Geometry check sheet. Reference: drawing and pictorial views, mm from the part's lowest x, y, z. A direction names the side the tool comes from. Give positions to 0.01 mm unless a question says otherwise; leave off trailing zeros. Order: outer loops, then holes, each group sorted by start corner. A loop starts at its lowest first (then second) coordinate and runs counter-clockwise, first axis right, second up. Notation, with made-up numbers: (-26, 61.25) - (25, 61.25) arc R29 cw to (25, 98.25) - close; hole circle Ø1 at (22, 46.5). An arc over 180 degrees is marked (long way). Answer as a JSON object with one key per item and string values.
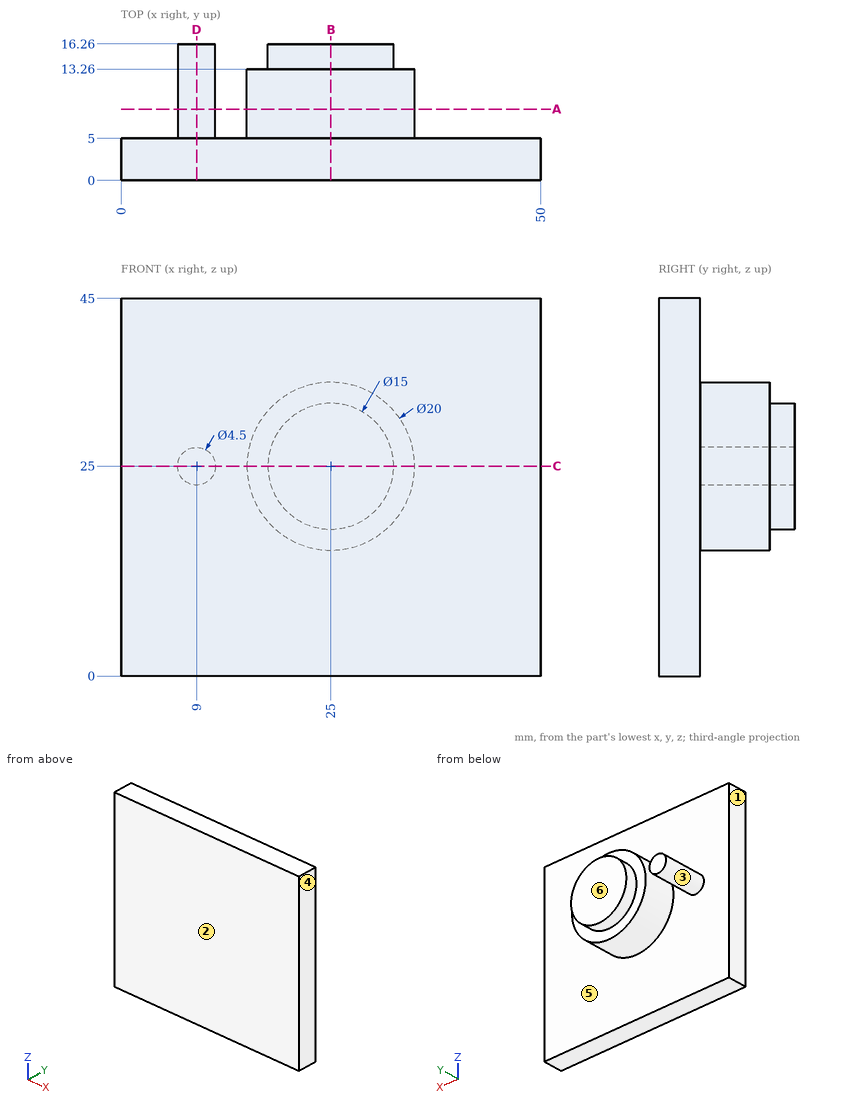
(1) Gauge pin test, flat ends, axial feed: pin 1 Ø6 at (x, y) = (35, 13) entering from -Z; pin 2 Ø1 at (x, y) = (8.5, 11) entering from +Z. Record the tip position at first contact, or that the pin passes through.
Computed values:
{"pin 1": "stops at z = 17.86", "pin 2": "stops at z = 27.25"}
(2) Section check B-B (x = 25). Record the cut outline in (y, z).
Computed values:
{"outline": "(0, 0) - (5, 0) - (5, 15) - (13.26, 15) - (13.26, 17.5) - (16.26, 17.5) - (16.26, 32.5) - (13.26, 32.5) - (13.26, 35) - (5, 35) - (5, 45) - (0, 45) - close"}
(3) Access from +Z, -Z, +X, -X, +Y, -Y to the whole of each face (thin tool, end or side, straight path). Record for the marked faces 5 and 6.
Computed values:
{"face 5": "+Y", "face 6": "+Z, -Z, +X, -X, +Y"}
(4) Section check C-C (z = 25). Record the cut outline in (x, y).
Computed values:
{"outline": "(0, 0) - (50, 0) - (50, 5) - (35, 5) - (35, 13.26) - (32.5, 13.26) - (32.5, 16.26) - (17.5, 16.26) - (17.5, 13.26) - (15, 13.26) - (15, 5) - (11.25, 5) - (11.25, 16.26) - (6.75, 16.26) - (6.75, 5) - (0, 5) - close"}
(5) Section check A-A (y = 8.5). Record the cut outline in (x, z).
Computed values:
{"outline": "circle Ø4.5 at (9, 25); circle Ø20 at (25, 25)"}
(6) Material ranges on line 1 along Y through (x, z) = (44.5, 43); line 2 along Y through (x, z) = (33.5, 30); line 3 along Z through (x, y) = (9, 9.5), recorded low to high. Write a range as [from, to].
Computed values:
{"line 1": "y = [0, 5]", "line 2": "y = [0, 13.26]", "line 3": "z = [22.75, 27.25]"}
(7) Section check D-D (x = 9). Record the cut outline in (y, z), then the cut area to 3 significant figures.
Computed values:
{"outline": "(0, 0) - (5, 0) - (5, 22.75) - (16.26, 22.75) - (16.26, 27.25) - (5, 27.25) - (5, 45) - (0, 45) - close", "area": "276 mm²"}
(8) Release check for a two-part mould opening along X. For the marked faces 1, 2, 3 and 4 record: pulls with the +X half, pulls with the -X half, needs draft (parallel to the pull), parting line crosses it, or undercut.
Computed values:
{"face 1": "pulls with the -X half", "face 2": "needs draft", "face 3": "undercut", "face 4": "pulls with the +X half"}
